from build123d import *

# Parameters (mm, degrees)
F0_R     = 1.6764
F0_W     = 5.842
F0_H     = 9.271
F1_DEPTH = 3.175


with BuildPart() as f1:
    # F0 (on Top) → F1 (new body)
    with BuildSketch(Plane.XY):
        with BuildLine():
            Line((34.223325677, 31.877), (-34.2168985559, 31.877))
            ThreePointArc((-34.2168985559, 31.877), (-35.9785916336, 32.4105870259), (-37.1481482894, 33.832))
            ThreePointArc((-37.1481482894, 33.832), (-45.4553961584, 35.0385567114), (-42.5824696374, 27.1510704541))
            ThreePointArc((-42.5824696374, 27.1510704541), (-40.7327787287, 26.0556077803), (-40.005, 24.0328045152))
            Line((-40.005, 24.0328045152), (-40.005, 18.161))
            Line((-40.005, 18.161), (-35.56, 18.161))
            Line((-35.56, 18.161), (-35.56, 27.178))
            Line((-35.56, 27.178), (-24.892, 27.178))
            Line((-24.892, 27.178), (-24.892, 4.445))
            Line((-24.892, 4.445), (-35.56, 4.445))
            Line((-35.56, 4.445), (-40.005, 4.445))
            Line((-40.005, 4.445), (-40.005, -12.827))
            Line((-40.005, -12.827), (-21.336, -12.827))
            Line((-21.336, -12.827), (-21.336, -23.749))
            Line((-21.336, -23.749), (-40.005, -23.749))
            Line((-40.005, -23.749), (-40.005, -24.0315756363))
            ThreePointArc((-40.005, -24.0315756363), (-40.7335995831, -26.0553715746), (-42.585, -27.1503253858))
            ThreePointArc((-42.585, -27.1503253858), (-45.4630746991, -35.0370175843), (-37.1545754104, -33.832))
            ThreePointArc((-37.1545754104, -33.832), (-35.9850187547, -32.4105870259), (-34.223325677, -31.877))
            Line((-34.223325677, -31.877), (34.223325677, -31.877))
            ThreePointArc((34.223325677, -31.877), (35.9850187547, -32.4105870259), (37.1545754104, -33.832))
            ThreePointArc((37.1545754104, -33.832), (45.4630746991, -35.0370175843), (42.585, -27.1503253858))
            ThreePointArc((42.585, -27.1503253858), (40.7335995831, -26.0553715746), (40.005, -24.0315756363))
            Line((40.005, -24.0315756363), (40.005, 24.0315756363))
            ThreePointArc((40.005, 24.0315756363), (40.7335995831, 26.0553715746), (42.585, 27.1503253858))
            ThreePointArc((42.585, 27.1503253858), (45.4630746991, 35.0370175843), (37.1545754104, 33.832))
            ThreePointArc((37.1545754104, 33.832), (35.9850187547, 32.4105870259), (34.223325677, 31.877))
        make_face()
        with Locations((-41.6687, -31.9532)):
            Circle(F0_R, mode=Mode.SUBTRACT)
        with BuildLine():
            Line((31.115, -27.051), (-7.239, -27.051))
            ThreePointArc((-7.239, -27.051), (-9.0350512242, -26.3070512242), (-9.779, -24.511))
            ThreePointArc((-9.779, -24.511), (-9.0350512242, -22.7149487758), (-7.239, -21.971))
            Line((-7.239, -21.971), (31.115, -21.971))
            ThreePointArc((31.115, -21.971), (32.9110512242, -22.7149487758), (33.655, -24.511))
            ThreePointArc((33.655, -24.511), (32.9110512242, -26.3070512242), (31.115, -27.051))
        make_face(mode=Mode.SUBTRACT)
        with Locations((41.6687, -31.9532)):
            Circle(F0_R, mode=Mode.SUBTRACT)
        with Locations((-41.6622728789, 31.9532)):
            Circle(F0_R, mode=Mode.SUBTRACT)
        with Locations((30.734, 2.6035)):
            Rectangle(F0_W, F0_H, mode=Mode.SUBTRACT)
        with BuildLine():
            Line((-21.209, 16.002), (-21.209, 27.178))
            Line((-21.209, 27.178), (30.988, 27.178))
            ThreePointArc((30.988, 27.178), (32.8738537854, 26.3968537854), (33.655, 24.511))
            ThreePointArc((33.655, 24.511), (32.8738537854, 22.6251462146), (30.988, 21.844))
            Line((30.988, 21.844), (-9.779, 21.844))
            Line((-9.779, 21.844), (-12.065, 21.844))
            Line((-12.065, 21.844), (-12.065, 16.002))
            Line((-12.065, 16.002), (-21.209, 16.002))
        make_face(mode=Mode.SUBTRACT)
        with Locations((41.6687, 31.9532)):
            Circle(F0_R, mode=Mode.SUBTRACT)
    extrude(amount=F1_DEPTH)


solid = f1.part
Verification items for the finished model (mm, model axes). A direction names the side the tool comes from. Give positions to 0.01 mm unless a question says otherwise; leave off trailing zeros. Write each loop counter-clockwise with the first axis right and the second up, starting at its lowest first coordinate (ties: lowest second). Pieces come first, ordered by that corner, then holes. Notation, with made-up numbers: (2, 65.25) -> (29, 65.25) arc R6 cw to (29, 69.25) -> close; hole circle Ø2 at (49, 77.5). An arc over 180 degrees is marked (long way). Use CSV: the item, a comma, the result in double quotes.
(1) Set-up check for faces 4 (the flat face through (40.005, 0, 2)), 5 (the flat face through (0, -31.877, 2)), 6 (the flat face through (-40.005, -4, 2)), 7 (the flat face through (10, 21.844, 2)): record each of +Z, -Z, +X, -X, +Y, -Y from which the full face is reachable in a straight line by a thin tool's end or side.
Derived:
face 4,"+Z, -Z, +X"
face 5,"+Z, -Z, -Y"
face 6,"+Z, -Z, -X"
face 7,"+Z, -Z"
(2) Material ranges on L1, parallel to Y at x = 2, z = 0.65; L2, parallel to Y at x = -25.5, z = 1.7 (3 decimals); L3, parallel to Y at x = -17, z = 0.55, recorded low to high.
Derived:
L1,"y = -31.88 to -27.05, -21.97 to 21.84, 27.18 to 31.88"
L2,"y = -31.877 to -23.749, -12.827 to 4.445, 27.178 to 31.877"
L3,"y = -31.88 to 16, 27.18 to 31.88"
(3) Sectioned sample at A-A (x = -26). Record the cut outline in (y, z) (3 decimals), plus the area to 3 significant figures.
Derived:
outline,"(-31.877, 0) -> (-23.749, 0) -> (-23.749, 3.175) -> (-31.877, 3.175) -> close; (-12.827, 0) -> (4.445, 0) -> (4.445, 3.175) -> (-12.827, 3.175) -> close; (27.178, 0) -> (31.877, 0) -> (31.877, 3.175) -> (27.178, 3.175) -> close"
area,"95.6 mm^2"
(4) Go/stop test with flat-tipped pins: pin 1 (1 mm diameter, centred on y = -10.5, z = 1, fed in from +X) (3 decimals); pin 2 (4 mm diameter, centred on x = 41.67, y = -31.95, fed in from +Z) (3 decimals); pin 3 (1.6 mm diameter, centred on x = -7.5, z = 1, fed in from +Y); pin 4 (1 mm diameter, centred on x = 14.5, z = 1, fed in from -Y). Record where each tip stops, or that it passes through.
Derived:
pin 1,"stops at x = 40.005"
pin 2,"stops at z = 3.175"
pin 3,"stops at y = 31.88"
pin 4,"stops at y = -31.88"
(5) Sectioned sample at D-D (z = 1.95). Give the number of separate pieces and of enclosed holes in the cut face, plus the area to 3 significant figures.
Derived:
separate pieces,"1"
enclosed holes,"7"
area,"4,220 mm^2"
(6) Sectioned sample at C-C (y = 14.5). Record the cut outline in (x, z) (3 decimals), plus the area to 3 significant figures.
Derived:
outline,"(-24.892, 0) -> (40.005, 0) -> (40.005, 3.175) -> (-24.892, 3.175) -> close"
area,"206 mm^2"
(7) Release check for a two-part mould opening along Y. For faces 1 (the cylindrical face through (35.963, -32.396, 1.565)), 2 (the flat face through (-1, 1, 3.175)), 3 (the flat face through (27.813, 3, 2)) record: +Y half, -Y half, draft (parallel to the pull), parting line (faces both ways), or undercut.
Derived:
face 1,"-Y half"
face 2,"draft"
face 3,"undercut"
(8) Sectioned sample at B-B (x = 4). Record the cut outline in (y, z) (3 decimals), plus the area to 3 significant figures.
Derived:
outline,"(-31.877, 0) -> (-27.051, 0) -> (-27.051, 3.175) -> (-31.877, 3.175) -> close; (-21.971, 0) -> (21.844, 0) -> (21.844, 3.175) -> (-21.971, 3.175) -> close; (27.178, 0) -> (31.877, 0) -> (31.877, 3.175) -> (27.178, 3.175) -> close"
area,"169 mm^2"
